The listing builds one solid part. Answer for the finished solid, in the listing's coordinates (mm). A direction names the side the tool comes from. Round coordinates to 2 decimals unless told otherwise and drop trailing zeros. Write each loop counter-clockwise with the first axis right and the second up, starting at its lowest first coordinate (ties: lowest second). Pieces come first, ordered by that corner, then holes.
Item 1: Find the intervals of material crossed by probe 1 along X at (y, z) = (60, 1.15); probe 2 along Y at (x, z) = (1.5, 30.5); probe 3 along Z at (x, y) = (-12.5, 62.25), in increasing order.
Item 2: Find section D-D on y = 60. Give the number of separate pieces and of enclosed holes in the cut face, then the cut area to 3 significant figures.
Item 3: For a pull along X with two mould halves and no side action, classify faces 1 (the face through (-2.32, 70.446, 2.225)), 2 (the face through (-21.5, 59.9, 2.2)), 3 (the face through (13, 58, 4)) as +X half, -X half, draft (parallel to the pull), parting line (faces both ways), or undercut.
Item 4: A tool of negligible diameter and unlimited length cuts with its end or side. For faces 4 (the face through (11.94, 52.13, 0.2)), 5 (the face through (-14.7, 58.7, 2)), from which of +Z, -Z, +X, -X, +Y, -Y can it reach the whole face along a straight path? Write none if from no direction.
Item 5: Find section A-A on x = 0. Give the vertices of the cut face in (y, z), then the cut area to 3 significant figures.
Item 6: Each of these flat-tipped pins is pushed along its axis until it touches: pin 1 (4 mm diameter, centred on x = 15.5, y = 56.5, fed in from +Z); pin 2 (8 mm diameter, centred on x = 0.5, z = 9, fed in from +Y); pin 3 (5 mm diameter, centred on x = 8, y = 58, fed in from -Z). Where does it stop, or does it pass through?
Item 7: Find section B-B on z = 15. Give the vertices of the cut face in (x, y), then the cut area to 3 significant figures.
Item 8: Find section C-C on x = -16. Give the vertices of the cut face in (y, z).
```python
from build123d import *

# Parameters (mm, degrees)
SKETCH020_R     = 10.7
SKETCH020_R_2   = 1.65
PAD001_DEPTH    = 4
SKETCH019_R     = 3
POCKET001_DEPTH = 2
CHAMFER001_SIZE = 0.4


with BuildPart() as part:
    # Sketch017 (on XZ_Plane004 of Origin010) → Revolution001 (revolve)
    with BuildSketch(Plane.XZ):
        with BuildLine():
            Line((7, 11), (6, 31))
            ThreePointArc((6, 31), (5.161048, 31.759052), (4.401996, 30.9201))
            Line((4.401996, 30.9201), (5.401996, 10.9201))
            ThreePointArc((5.401996, 10.9201), (5.654041, 9.857767), (6.269565, 8.955986))
            Line((10.351475, 4.845571), (6.269565, 8.955986))
            ThreePointArc((10.7, 4), (10.609453, 4.457291), (10.351475, 4.845571))
            Line((10.7, 4), (12.5, 4))
            ThreePointArc((12.5, 4), (12.253216, 5.191554), (11.553466, 6.187071))
            Line((11.553466, 6.187071), (7.439969, 10.04928))
            ThreePointArc((7, 11), (7.127708, 10.481937), (7.439969, 10.04928))
        make_face()
    revolve(axis=Axis((0, 0, 0), (0, 0, 1)))

    # Sketch020 (on Face1 of Revolution001) → Pad001 (new body)
    with BuildSketch(Plane(origin=(0, 0, 4), x_dir=(1, 0, 0), z_dir=(0, 0, -1))):
        with BuildLine():
            ThreePointArc((5.46875, 11.24023), (0, 12.5), (-5.46875, 11.24023))
            Line((-5.46875, 11.24023), (-18.40625, 4.945701))
            ThreePointArc((-18.40625, 4.945701), (-21.5, 0), (-18.40625, -4.945701))
            Line((-18.40625, -4.945701), (-5.46875, -11.24023))
            ThreePointArc((-5.46875, -11.24023), (0, -12.5), (5.46875, -11.24023))
            Line((5.46875, -11.24023), (18.40625, -4.945701))
            ThreePointArc((18.40625, -4.945701), (21.5, 0), (18.40625, 4.945701))
            Line((5.46875, 11.24023), (18.40625, 4.945701))
        make_face()
        Circle(SKETCH020_R, mode=Mode.SUBTRACT)
        with Locations((-16, 0)):
            Circle(SKETCH020_R_2, mode=Mode.SUBTRACT)
        with Locations((16, 0)):
            Circle(SKETCH020_R_2, mode=Mode.SUBTRACT)
    extrude(amount=PAD001_DEPTH)

    # Sketch019 (on Face3 of Pad001) → Pocket001 (cut)
    with BuildSketch(Plane.XY.offset(4)):
        with Locations((-16, 0)):
            Circle(SKETCH019_R)
        with Locations((16, 0)):
            Circle(SKETCH019_R)
    extrude(amount=-POCKET001_DEPTH, mode=Mode.SUBTRACT)

    # Chamfer001
    chamfer001_edges = [part.edges().sort_by_distance(p)[0] for p in [
        (-10.7, 0, 0),
        (-17.65, 0, 0),
        (14.35, 0, 0),
        (-11.9375, 8.092966, 0),
    ]]
    chamfer(chamfer001_edges, length=CHAMFER001_SIZE)


with BuildPart() as part_1:
    # Body004 placement: moved
    add(part.part.moved(Location((0, 60, 0))))


solid = part_1.part
```
Check values:
1. probe 1: x = -21.5 to -17.65, -14.35 to -10.7, 10.7 to 14.35, 17.65 to 21.5
1. probe 2: y = 54.16 to 55.84, 64.16 to 65.84
1. probe 3: z = 0 to 4
2. separate pieces: 4
2. enclosed holes: 0
2. area: 145 mm2
3. face 1: undercut
3. face 2: -X half
3. face 3: draft
4. face 4: -Z, +X, -Y
4. face 5: +Z
5. outline: (47.5, 0.4) - (47.9, 0) - (48.9, 0) - (49.3, 0.4) - (49.3, 4) arc R1.2 cw to (49.65, 4.85) - (53.73, 8.96) arc R3 ccw to (54.6, 10.92) - (55.6, 30.92) arc R0.8 ccw to (54, 31) - (53, 11) arc R1.4 cw to (52.56, 10.05) - (48.45, 6.19) arc R3 ccw to (47.5, 4) - close; (64.4, 30.92) - (65.4, 10.92) arc R3 ccw to (66.27, 8.96) - (70.35, 4.85) arc R1.2 cw to (70.7, 4) - (70.7, 0.4) - (71.1, 0) - (72.1, 0) - (72.5, 0.4) - (72.5, 4) arc R3 ccw to (71.55, 6.19) - (67.44, 10.05) arc R1.4 cw to (67, 11) - (66, 31) arc R0.8 ccw to start
5. area: 111 mm2
6. pin 1: stops at z = 4
6. pin 2: stops at y = 72.32
6. pin 3: stops at z = 0.35
7. outline: circle Ø13.6 at (0, 60); hole circle Ø10.4 at (0, 60)
7. area: 60.4 mm2
8. outline: (53.88, 0.4) - (54.33, 0) - (57.95, 0) - (58.35, 0.4) - (58.35, 2) - (57, 2) - (57, 4) - (53.88, 4) - close; (61.65, 0.4) - (62.05, 0) - (65.67, 0) - (66.12, 0.4) - (66.12, 4) - (63, 4) - (63, 2) - (61.65, 2) - close
